CAD build for the part. Positions are in the model's coordinates, mm. Face numbers are marked on the shaded views. A direction names the side the tool comes from. Round coordinates to 2 decimals unless told otherwise and drop trailing zeros. Loops run counter-clockwise (first coordinate to the right, second up) from the corner with the lowest first, then second, coordinate; pieces in that order, holes last. Notation, with made-up numbers: (-32.5, -26) - (-20.5, -26) arc R28 cw to (-20.5, -3) - close; hole circle Ø3 at (66, 65). An arc over 180 degrees is marked (long way). One line per question, with ' | ' between items.
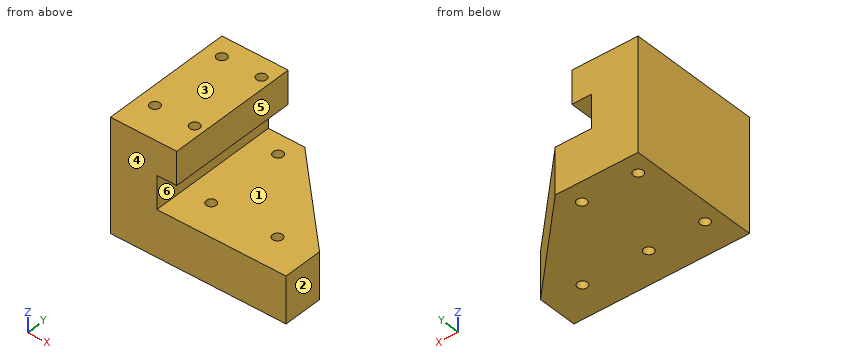
```python
from build123d import *

# Parameters (mm, degrees)
SKETCH_1_W          = 20
SKETCH_1_H          = 40
EXTRUDE_1_DEPTH     = 34
SKETCH_2_R          = 1.5
CUT_EXTRUDE_1_DEPTH = 57.178287621
EXTRUDE_START       = -34
SKETCH_3_W          = 33
SKETCH_3_H          = 40
EXTRUDE_2_DEPTH     = 14
CUT_EXTRUDE_2_DEPTH = 75.598927606
SKETCH_5_R          = 1.5
CUT_EXTRUDE_3_DEPTH = 75.598927606
SKETCH_6_W          = 6
SKETCH_6_H          = 10
CUT_EXTRUDE_4_DEPTH = 75.598927606
SKETCH_7_R          = 1.5
CUT_EXTRUDE_5_DEPTH = 10


with BuildPart() as part:
    # 草图1 → 凸台-拉伸1 (new body)
    with BuildSketch(Plane.XY):
        with Locations((10, 20)):
            Rectangle(SKETCH_1_W, SKETCH_1_H)
    extrude(amount=EXTRUDE_1_DEPTH)

    # 草图2 → 切除-拉伸1 (cut, through all)
    with BuildSketch(Plane.XY.offset(34)):
        with Locations((5, 34)):
            Circle(SKETCH_2_R)
        with Locations((5, 10)):
            Circle(SKETCH_2_R)
    extrude(amount=-CUT_EXTRUDE_1_DEPTH, mode=Mode.SUBTRACT)

    # 草图3 → 凸台-拉伸2 (add)
    with BuildSketch(Plane.XY.offset(34).offset(EXTRUDE_START)):
        with Locations((36.5, 20)):
            Rectangle(SKETCH_3_W, SKETCH_3_H)
    extrude(amount=EXTRUDE_2_DEPTH)

    # 草图4 → 切除-拉伸2 (cut, through all)
    with BuildSketch(Plane(origin=(0, 0, 0), x_dir=(-1, 0, 0), z_dir=(0, 0, -1))):
        Polygon((-25, 40), (-53, 40), (-53, 12), align=None)
    extrude(amount=-CUT_EXTRUDE_2_DEPTH, mode=Mode.SUBTRACT)

    # 草图5 → 切除-拉伸3 (cut, through all)
    with BuildSketch(Plane(origin=(0, 0, 0), x_dir=(-1, 0, 0), z_dir=(0, 0, -1))):
        with Locations((-22, 34)):
            Circle(SKETCH_5_R)
        with Locations((-22, 10)):
            Circle(SKETCH_5_R)
        with Locations((-42, 10)):
            Circle(SKETCH_5_R)
    extrude(amount=-CUT_EXTRUDE_3_DEPTH, mode=Mode.SUBTRACT)

    # 草图6 → 切除-拉伸4 (cut, through all)
    with BuildSketch(Plane.XZ):
        with Locations((17, 19)):
            Rectangle(SKETCH_6_W, SKETCH_6_H)
    extrude(amount=-CUT_EXTRUDE_4_DEPTH, mode=Mode.SUBTRACT)

    # 草图7 → 切除-拉伸5 (cut)
    with BuildSketch(Plane.XY.offset(34)):
        with Locations((17, 34)):
            Circle(SKETCH_7_R)
        with Locations((17, 10)):
            Circle(SKETCH_7_R)
    extrude(amount=-CUT_EXTRUDE_5_DEPTH, mode=Mode.SUBTRACT)


solid = part.part
```
(1) Drop flat-ended pins along their axis: P1, Ø5, axis at y = 22.5, z = 17.5, coming from the +X side; P2, Ø11.5, axis at x = 34, y = 11, coming from the +Z side; P3, Ø1, axis at y = 26.5, z = 30, coming from the +X side; P4, Ø2.5, axis at x = 5, y = 34, coming from the -Z side. Give the stop position or say it passes through.
Results found:
P1: stops at x = 14 | P2: stops at z = 14 | P3: stops at x = 20 | P4: passes through
(2) Cut at B-B, the plane y = 10. Write the cut outline in (x, z).
Results found:
outline: (0, 0) - (3.5, 0) - (3.5, 34) - (0, 34) - close; (6.5, 0) - (20.5, 0) - (20.5, 14) - (14, 14) - (14, 24) - (15.5, 24) - (15.5, 34) - (6.5, 34) - close; (18.5, 24) - (20, 24) - (20, 34) - (18.5, 34) - close; (23.5, 0) - (40.5, 0) - (40.5, 14) - (23.5, 14) - close; (43.5, 0) - (53, 0) - (53, 14) - (43.5, 14) - close
(3) Two-plate mould, pull along Z, no slides. Class the marked faces 1, 2 and 3: released by +Z, released by -Z, zero draft, split by the parting line, or undercut.
Results found:
face 1: undercut | face 2: zero draft | face 3: released by +Z
(4) Tool access for the marked faces 4, 5 and 6: list every direction of +Z, -Z, +X, -X, +Y, -Y with a clear straight run to the whole face (end or side of a thin tool).
Results found:
face 4: +Z, -Z, +X, -X, -Y | face 5: +Z, +X, +Y, -Y | face 6: +X, +Y, -Y
(5) Cut at D-D, the plane z = 28. Write the cut outline in (x, y).
Results found:
outline: (0, 0) - (20, 0) - (20, 40) - (0, 40) - close; hole circle Ø3 at (5, 10); hole circle Ø3 at (5, 34); hole circle Ø3 at (17, 10); hole circle Ø3 at (17, 34)
(6) Cut at C-C, the plane x = 5. Write the cut outline in (y, z), then the cut area to 3 significant figures.
Results found:
outline: (0, 0) - (8.5, 0) - (8.5, 34) - (0, 34) - close; (11.5, 0) - (32.5, 0) - (32.5, 34) - (11.5, 34) - close; (35.5, 0) - (40, 0) - (40, 34) - (35.5, 34) - close | area: 1,160 mm²
(7) Probe L1, parallel to Y at x = 5, z = 23; L2, parallel to Z at x = 18, y = 2; L3, parallel to X at y = 9.5, z = 11. List the from-to ranges inside material, lowest first.
Results found:
L1: y = 0 to 8.5, 11.5 to 32.5, 35.5 to 40 | L2: z = 0 to 14, 24 to 34 | L3: x = 0 to 3.59, 6.41 to 20.59, 23.41 to 40.59, 43.41 to 53
(8) Cut at A-A, the plane x = 17. Write the cut outline in (y, z).
Results found:
outline: (0, 0) - (40, 0) - (40, 14) - (0, 14) - close; (0, 24) - (8.5, 24) - (8.5, 34) - (0, 34) - close; (11.5, 24) - (32.5, 24) - (32.5, 34) - (11.5, 34) - close; (35.5, 24) - (40, 24) - (40, 34) - (35.5, 34) - close
